Geometry: final body of the model. Coordinates: model frame, mm. Give positions to 0.01 mm unless a question says otherwise; leave off trailing zeros. Answer as a JSON object with one key per item and string values. Group by question number.
(1) Contact query for flat-ended pins moving along their axis: pin 1 Ø0.9 at (x, z) = (34.5, -6.5) entering from -Y; pin 2 Ø0.9 at (x, z) = (-15, -6.5) entering from +Y; pin 3 Ø0.5 at (x, z) = (-14.5, -6) entering from -Y. Output: stop coordinate, or through.
(2) Draft query along X for faces 1 (the face through (1, -1, -7)), 2 (the face through (-22.09, -23.22, -6.11)). Return one class per face: +X half, -X half, draft (parallel to the pull), parting line (faces both ways), or undercut.
(3) Section query A-A on x = 20. State how many separate pieces and enclosed holes the cut face has, plus the area to 3 significant figures.
(4) Material intervals for probe 1 along X at (y, z) = (29.5, -5.35); probe 2 along Y at (x, z) = (-36, -6.65); probe 3 along X at (y, z) = (-18, -6.1), sorted ascending.
from build123d import *

# Parameters (mm, degrees)
POCKET004_DEPTH       = 234.354933
POLARPATTERN001_COUNT = 8


with BuildPart() as part:
    # Sketch017 → Revolution (revolve)
    with BuildSketch(Plane.XZ):
        Polygon((-40.35, -5.2), (-41.10519, -6.1), (-40.35, -7), (0, -7), (0, -5.2), align=None)
    revolve(axis=Axis((0, 0, 0), (0, 0, 1)))

    # Sketch018 → Pocket004 (cut, through all)
    with BuildSketch(Plane.XY.offset(-7)):
        with BuildLine():
            Line((0.8, 9.967949), (0.8, 23.679871))
            ThreePointArc((16.178512, 17.309883), (9.067064, 21.88983), (0.8, 23.679871))
            Line((6.482719, 7.614089), (16.178512, 17.309883))
            ThreePointArc((6.482719, 7.614089), (3.826834, 9.238795), (0.8, 9.967949))
        make_face()
        with BuildLine():
            ThreePointArc((17.309883, 18.441254), (9.679031, 23.367248), (0.8, 25.279871))
            Line((0.8, 25.279871), (0.8, 38.991794))
            ThreePointArc((27.005677, 28.137047), (14.924654, 36.031302), (0.8, 38.991794))
            Line((17.309883, 18.441254), (27.005677, 28.137047))
        make_face()
    pocket004 = extrude(amount=POCKET004_DEPTH, mode=Mode.SUBTRACT)

    # PolarPattern001: Pocket004 ×8 about axis
    polarpattern001_axis = Axis((0, 0, -7), (0, 0, 1))
    for i in range(1, POLARPATTERN001_COUNT):
        add(pocket004.rotate(polarpattern001_axis, i * 360 / POLARPATTERN001_COUNT), mode=Mode.SUBTRACT)


solid = part.part
Answer list:
{
 "1": {"pin 1": "y = -22.71", "pin 2": "y = 38.35", "pin 3": "y = -38.55"},
 "2": {"face 1": "draft", "face 2": "undercut"},
 "3": {"separate pieces": "7", "enclosed holes": "0", "area": "28.2 mm2"},
 "4": {"probe 1": "-27.71 to -25.51, -0.8 to 0.8, 25.51 to 27.71", "probe 2": "-18.87 to -15, -0.8 to 0.8, 15 to 18.87", "probe 3": "-36.95 to -34.6, -19.13 to -15.41, -0.8 to 0.8, 15.41 to 19.13, 34.6 to 36.95"}
}
